```python
from build123d import *

# Parameters (mm, degrees)
XOR_EXTRUDE1_580_DEPTH          = 11
XOR_EXTRUDE1_580_DEPTH_BACK     = 8.5
XOR_EXTRUDE2_CUT_582_DEPTH      = 23
XOR_EXTRUDE3_CUT_585_DEPTH      = 30
XOR_EXTRUDE3_CUT_585_DEPTH_BACK = 31.5
XOR_SKETCH4_MESH_586_R          = 2
XOR_EXTRUDE4_CUT_587_DEPTH      = 30
XOR_SKETCH5_MESH_588_R          = 3.4
XOR_EXTRUDE5_CUT_949_DEPTH      = 1
XOR_SKETCH6_MESH_1066_W         = 3.25
XOR_SKETCH6_MESH_1066_H         = 5
XOR_SKETCH6_MESH_1066_W_2       = 2.9
XOR_EXTRUDE6_MERGE_1279_DEPTH   = 2
XOR_SKETCH7_MESH_2256_W         = 3
XOR_SKETCH7_MESH_2256_H         = 3.62350981
XOR_EXTRUDE7_CUT_2327_DEPTH     = 4


with BuildPart() as part:
    # XOR_Sketch1 (Mesh)_7 → XOR_Extrude1_580 (new, two sides: drawn at the far end of the back side and taken through both)
    with BuildSketch(Plane.XY.offset(-XOR_EXTRUDE1_580_DEPTH_BACK)):
        with BuildLine():
            Line((11.901247371, 18.104240693), (-12.098752629, 18.104240693))
            ThreePointArc((-12.098752629, 18.104240693), (-13.512966192, 18.690027131), (-14.098752629, 20.104240693))
            Line((-14.098752629, 20.104240693), (-14.098752629, 25.104240693))
            Line((-14.098752629, 25.104240693), (-34.098752629, 25.104240693))
            ThreePointArc((-34.098752629, 25.104240693), (-38.341393316, 23.34688138), (-40.098752629, 19.104240693))
            Line((-40.098752629, 19.104240693), (-40.098752629, -18.895759307))
            ThreePointArc((-40.098752629, -18.895759307), (-38.341393316, -23.138399994), (-34.098752629, -24.895759307))
            Line((-34.098752629, -24.895759307), (-14.098752629, -24.895759307))
            Line((-14.098752629, -24.895759307), (-14.098752629, -21.570783007))
            ThreePointArc((-14.098752629, -21.570783007), (-13.512966192, -20.156569445), (-12.098752629, -19.570783007))
            Line((-12.098752629, -19.570783007), (11.901247371, -19.570783007))
            ThreePointArc((11.901247371, -19.570783007), (13.315460933, -20.156569445), (13.901247371, -21.570783007))
            Line((13.901247371, -21.570783007), (13.901247371, -24.895759307))
            Line((13.901247371, -24.895759307), (33.901247371, -24.895759307))
            ThreePointArc((33.901247371, -24.895759307), (38.143888058, -23.138399994), (39.901247371, -18.895759307))
            Line((39.901247371, -18.895759307), (39.901247371, 19.104240693))
            ThreePointArc((39.901247371, 19.104240693), (38.143888058, 23.34688138), (33.901247371, 25.104240693))
            Line((33.901247371, 25.104240693), (13.901247371, 25.104240693))
            Line((13.901247371, 25.104240693), (13.901247371, 20.104240693))
            ThreePointArc((13.901247371, 20.104240693), (13.315460933, 18.690027131), (11.901247371, 18.104240693))
        make_face()
    extrude(amount=XOR_EXTRUDE1_580_DEPTH + XOR_EXTRUDE1_580_DEPTH_BACK)

    # XOR_Sketch2 (Mesh)_581 → XOR_Extrude2 (Cut)_582 (cut)
    with BuildSketch(Plane.XY):
        with BuildLine():
            Line((37.042591497, 18.002105269), (37.042591497, -14.420226453))
            ThreePointArc((37.042591497, -14.420226453), (36.027448956, -17.267289587), (33.440027724, -18.829830542))
            ThreePointArc((33.440027724, -18.829830542), (16.804364648, -21.403203006), (0, -22.393587061))
            ThreePointArc((0, -22.393587061), (-16.804364648, -21.403203006), (-33.440027724, -18.829830542))
            ThreePointArc((-33.440027724, -18.829830542), (-36.027448956, -17.267289587), (-37.042591497, -14.420226453))
            Line((-37.042591497, -14.420226453), (-37.042591497, 18.002105269))
            ThreePointArc((-37.042591497, 18.002105269), (-35.772866321, 21.135047107), (-32.680225027, 22.5))
            Line((-32.680225027, 22.5), (0, 23.5))
            Line((0, 23.5), (32.680225027, 22.5))
            ThreePointArc((32.680225027, 22.5), (35.772866321, 21.135047107), (37.042591497, 18.002105269))
        make_face()
    extrude(amount=XOR_EXTRUDE2_CUT_582_DEPTH, mode=Mode.SUBTRACT)

    # XOR_Sketch3 (Mesh)_583 → XOR_Extrude3 (Cut)_585 (cut, two sides: drawn at the far end of the back side and taken through both)
    with BuildSketch(Plane(origin=(0, 0, 0), x_dir=(1, 0, 0), z_dir=(0, 1, 0)).offset(-XOR_EXTRUDE3_CUT_585_DEPTH_BACK)):
        with BuildLine():
            Line((35, -7), (35, -20.680063706))
            Line((35, -20.680063706), (45.656007765, -20.680063706))
            Line((45.656007765, -20.680063706), (45.656007765, -6.5))
            Line((45.656007765, -6.5), (35.5, -6.5))
            ThreePointArc((35.5, -6.5), (35.146446609, -6.646446609), (35, -7))
        make_face()
        with BuildLine():
            Line((-45.656007765, -20.680063706), (-45.656007765, -6.5))
            Line((-45.656007765, -6.5), (-35.5, -6.5))
            ThreePointArc((-35.5, -6.5), (-35.146446609, -6.646446609), (-35, -7))
            Line((-35, -7), (-35, -20.680063706))
            Line((-35, -20.680063706), (-45.656007765, -20.680063706))
        make_face()
    extrude(amount=XOR_EXTRUDE3_CUT_585_DEPTH + XOR_EXTRUDE3_CUT_585_DEPTH_BACK, mode=Mode.SUBTRACT)

    # XOR_Sketch4 (Mesh)_586 → XOR_Extrude4 (Cut)_587 (cut)
    with BuildSketch(Plane.XY):
        with Locations((-17, -17)):
            Circle(XOR_SKETCH4_MESH_586_R)
        with Locations((-17, 17)):
            Circle(XOR_SKETCH4_MESH_586_R)
        with Locations((17, -17)):
            Circle(XOR_SKETCH4_MESH_586_R)
        with Locations((17, 17)):
            Circle(XOR_SKETCH4_MESH_586_R)
    extrude(amount=-XOR_EXTRUDE4_CUT_587_DEPTH, mode=Mode.SUBTRACT)

    # XOR_Sketch5 (Mesh)_588 → XOR_Extrude5 (Cut)_949 (cut)
    with BuildSketch(Plane.XY):
        with Locations((16.910776866, 17.14358453)):
            Circle(XOR_SKETCH5_MESH_588_R)
        with Locations((-17.089223134, 17.14358453)):
            Circle(XOR_SKETCH5_MESH_588_R)
        with Locations((16.910776866, -16.85641547)):
            Circle(XOR_SKETCH5_MESH_588_R)
        with Locations((-17.089223134, -16.85641547)):
            Circle(XOR_SKETCH5_MESH_588_R)
    extrude(amount=-XOR_EXTRUDE5_CUT_949_DEPTH, mode=Mode.SUBTRACT)

    # XOR_Sketch6 (Mesh)_1066 → XOR_Extrude6 (Merge)_1279 (add)
    with BuildSketch(Plane.XY.offset(6.5)):
        with Locations((-36.625, -7.5)):
            Rectangle(XOR_SKETCH6_MESH_1066_W, XOR_SKETCH6_MESH_1066_H)
        with Locations((-36.45, 12.5)):
            Rectangle(XOR_SKETCH6_MESH_1066_W_2, XOR_SKETCH6_MESH_1066_H)
    extrude(amount=-XOR_EXTRUDE6_MERGE_1279_DEPTH)

    # XOR_Sketch7 (Mesh)_2256 → XOR_Extrude7 (Cut)_2327 (cut)
    with BuildSketch(Plane.XY.offset(6.5)):
        with Locations((-36.5, 6.311754905)):
            Rectangle(XOR_SKETCH7_MESH_2256_W, XOR_SKETCH7_MESH_2256_H)
    extrude(amount=-XOR_EXTRUDE7_CUT_2327_DEPTH, mode=Mode.SUBTRACT)


solid = part.part
```
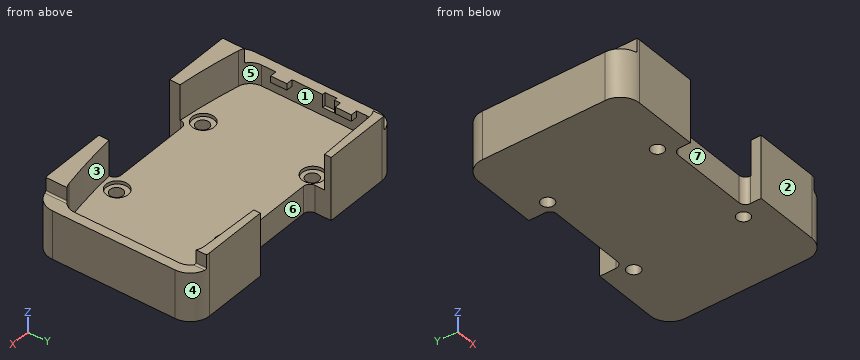
Source: CAD feature listing. Evaluate the final solid. Frame: model axes, mm. Face numbers are marked on the shaded views. A direction names the side the tool comes from. Give positions to 0.01 mm unless a question says otherwise; leave off trailing zeros. Loops run counter-clockwise (first coordinate to the right, second up) from the corner with the lowest first, then second, coordinate; pieces in that order, holes last. Notation, with made-up numbers: (39.5, 76.25) - (90.5, 76.25) arc R11 ccw to (90.5, 89.25) - close; hole circle Ø8 at (-20, 33.5). An arc over 180 degrees is marked (long way). Use CSV: the item, a comma, the result in double quotes. Start each with the question number.
1. Reachability of the marked faces 5, 6 and 7 from +Z, -Z, +X, -X, +Y, -Y: full face, straight path, thin tool, end or side. Return the list, or none.
2. Section A-A (z = -6.5). Output: boundary loops of the cut face in (x, y), then the cut area to 3 significant figures.
3. Section D-D (x = 28.5). Output: boundary loops of the cut face in (y, z).
4. Section C-C (x = 6.5). Output: boundary loops of the cut face in (y, z).
5. Ray query, L1, parallel to Y at x = -17, z = -0.5; L2, parallel to Y at x = -17, z = -4.25; L3, parallel to X at y = -1.5, z = 3.75. Return the intervals inside material, ascending.
6. Pin query (flat end, axial travel): pin 1 (10 mm diameter, centred on x = -8.5, y = 16.5, fed in from +Z); pin 2 (5.5 mm diameter, centred on y = 22, z = 5.5, fed in from +X); pin 3 (4 mm diameter, centred on x = -17.09, y = 17.14, fed in from -Z); pin 4 (9.5 mm diameter, centred on x = -1, z = -3.5, fed in from -Y). Return the tip coordinate at first contact, or that it passes through.
7. Draft query along X for the marked faces 1, 2, 3 and 4. Return one class per face: +X half, -X half, draft (parallel to the pull), parting line (faces both ways), or undercut.
8. Section B-B (x = 17). Output: boundary loops of the cut face in (y, z).
Response:
1,face 5,"+Z"
1,face 6,"+Z, -Z, +Y"
1,face 7,"+Z, -Z, -Y"
2,outline,"(-40.1, -18.9) arc R6 ccw to (-34.1, -24.9) - (-14.1, -24.9) - (-14.1, -21.57) arc R2 cw to (-12.1, -19.57) - (11.9, -19.57) arc R2 cw to (13.9, -21.57) - (13.9, -24.9) - (33.9, -24.9) arc R6 ccw to (39.9, -18.9) - (39.9, 19.1) arc R6 ccw to (33.9, 25.1) - (13.9, 25.1) - (13.9, 20.1) arc R2 cw to (11.9, 18.1) - (-12.1, 18.1) arc R2 cw to (-14.1, 20.1) - (-14.1, 25.1) - (-34.1, 25.1) arc R6 ccw to (-40.1, 19.1) - close; hole circle Ø4 at (-17, -17); hole circle Ø4 at (-17, 17); hole circle Ø4 at (17, -17); hole circle Ø4 at (17, 17)"
2,area,"3,580 mm²"
3,outline,"(-24.9, -8.5) - (25.1, -8.5) - (25.1, 11) - (22.63, 11) - (22.63, 0) - (-19.76, 0) - (-19.76, 11) - (-24.9, 11) - close"
4,outline,"(-19.57, -8.5) - (18.1, -8.5) - (18.1, 0) - (-19.57, 0) - close"
5,L1,"-24.9 to -20.26, -13.46 to 13.74, 20.54 to 25.1"
5,L2,"-24.9 to -19, -15 to 15, 19 to 25.1"
5,L3,"-40.1 to -37.04, 37.04 to 39.9"
6,pin 1,"z = 0"
6,pin 2,"x = 39.9"
6,pin 3,"z = -8.5"
6,pin 4,"y = -19.57"
7,face 1,"undercut"
7,face 2,"draft"
7,face 3,"undercut"
7,face 4,"+X half"
8,outline,"(-24.9, -8.5) - (-19, -8.5) - (-19, -1) - (-20.26, -1) - (-20.26, 0) - (-21.38, 0) - (-21.38, 11) - (-24.9, 11) - close; (-15, -8.5) - (15, -8.5) - (15, -1) - (13.74, -1) - (13.74, 0) - (-13.46, 0) - (-13.46, -1) - (-15, -1) - close; (19, -8.5) - (25.1, -8.5) - (25.1, 11) - (22.98, 11) - (22.98, 0) - (20.54, 0) - (20.54, -1) - (19, -1) - close"
